from build123d import *

# Parameters (mm, degrees)
BOSS_EXTRUDE1_DEPTH = 13
SKETCH1_3_W         = 30
SKETCH1_3_H         = 13
BOSS_EXTRUDE2_DEPTH = 37
SKETCH2_R           = 8
CUT_EXTRUDE1_DEPTH  = 37


with BuildPart() as part:
    # Sketch1 → Boss-Extrude1 (new body)
    with BuildSketch(Plane(origin=(0, 0, 0), x_dir=(1, 0, 0), z_dir=(0, 1, 0))):
        with BuildLine():
            ThreePointArc((0, 30), (-15, 15), (0, 0))
            Line((0, 0), (0, 8.5))
            ThreePointArc((0, 8.5), (-6.5, 15), (0, 21.5))
            Line((0, 21.5), (0, 30))
        make_face()
        with BuildLine():
            Line((0, 8.5), (0, 0))
            ThreePointArc((0, 0), (10.606601718, 4.393398282), (15, 15))
            ThreePointArc((15, 15), (10.606601718, 25.606601718), (0, 30))
            Line((0, 30), (0, 21.5))
            ThreePointArc((0, 21.5), (4.596194078, 19.596194078), (6.5, 15))
            ThreePointArc((6.5, 15), (4.596194078, 10.403805922), (0, 8.5))
        make_face()
        with BuildLine():
            ThreePointArc((15, 15), (10.606601718, 4.393398282), (0, 0))
            Line((0, 0), (35, 0))
            Line((35, 0), (35, 30))
            Line((35, 30), (5, 30))
            Line((5, 30), (0, 30))
            ThreePointArc((0, 30), (10.606601718, 25.606601718), (15, 15))
        make_face()
    extrude(amount=BOSS_EXTRUDE1_DEPTH)

    # Sketch1_3 → Boss-Extrude2 (add)
    with BuildSketch(Plane(origin=(0, 0, 0), x_dir=(1, 0, 0), z_dir=(0, 1, 0))):
        with Locations((20, 36.5)):
            Rectangle(SKETCH1_3_W, SKETCH1_3_H)
    extrude(amount=BOSS_EXTRUDE2_DEPTH)

    # Sketch2 → Cut-Extrude1 (cut)
    with BuildSketch(Plane.XY.offset(-30)):
        with Locations((20, 25)):
            Circle(SKETCH2_R)
    extrude(amount=-CUT_EXTRUDE1_DEPTH, mode=Mode.SUBTRACT)


solid = part.part
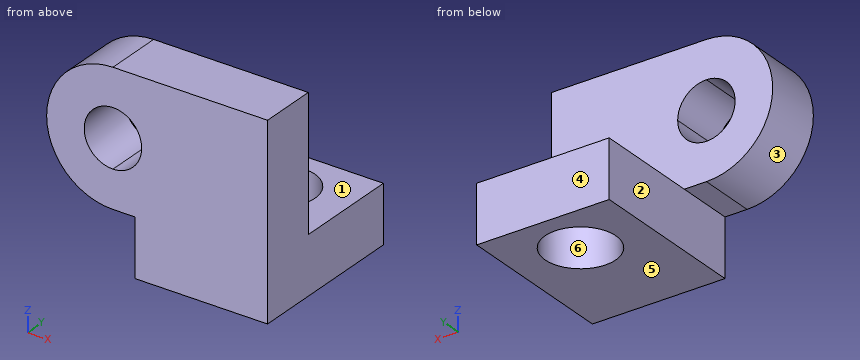
Part model, mm, in its own coordinate system. Face numbers are marked on the shaded views. A direction names the side the tool comes from. Coordinates: 2 decimals unless noted, no trailing zeros. Order: outer loops, then holes, each group sorted by start corner. A loop starts at its lowest first (then second) coordinate and runs counter-clockwise, first axis right, second up. Notation, with made-up numbers: M 63,23.5 L 112,23.5 A35 cw 112,60.5 Z; hole C 54,82.25 d5. An arc over 180 degrees is marked long. Use a Markdown table: item, result.
(1) Flat gauge pins, fed straight in: pin 1 (14.5 mm diameter, centred on x = 20, y = 25, fed in from +Z); pin 2 (10 mm diameter, centred on x = 2, y = 18.5, fed in from +Z); pin 3 (10 mm diameter, centred on x = 3, z = -19, fed in from +Y); pin 4 (6.5 mm diameter, centred on y = 16, z = -33.5, fed in from -X). Where does each tip first touch, or does it go through?
A:
| item | result |
|---|---|
| pin 1 | passes through |
| pin 2 | stops at z = -30 |
| pin 3 | stops at y = 13 |
| pin 4 | stops at x = 5 |
(2) Probe L1, parallel to Y at x = 20, z = -38; L2, parallel to Y at x = 4.5, z = -23; L3, parallel to Z at x = -2.5, y = 5. List the from-to ranges inside material, lowest first.
A:
| item | result |
|---|---|
| L1 | y = 0 to 17, 33 to 37 |
| L2 | y = 0 to 13 |
| L3 | z = -29.79 to -21, -9 to -0.21 |
(3) Cut at B-B on y = 7. Write the cut outline in (x, z), then the cut area to 3 significant figures.
A:
| item | result |
|---|---|
| outline | M 0,-30 L 5,-30 L 5,-43 L 35,-43 L 35,0 L 0,0 A15 ccw Z; hole C 0,-15 d13 |
| area | 1,660 mm^2 |
(4) Cut at A-A on x = 20. Write the cut outline in (y, z).
A:
| item | result |
|---|---|
| outline | M 0,-43 L 17,-43 L 17,-30 L 13,-30 L 13,0 L 0,0 Z; M 33,-43 L 37,-43 L 37,-30 L 33,-30 Z |
(5) Cut at D-D on x = 31.5. Write the cut outline in (y, z), then the cut area to 3 significant figures.
A:
| item | result |
|---|---|
| outline | M 0,-43 L 37,-43 L 37,-30 L 13,-30 L 13,0 L 0,0 Z |
| area | 871 mm^2 |
(6) Pull direction Y, two halves, no side cores. Call the marked faces 4, 5 and 6: released by +Y, released by -Y, zero draft, split by the parting line, or undercut.
A:
| item | result |
|---|---|
| face 4 | released by +Y |
| face 5 | zero draft |
| face 6 | undercut |
(7) Cut at C-C on z = -33. Write the cut outline in (x, y).
A:
| item | result |
|---|---|
| outline | M 5,0 L 35,0 L 35,37 L 5,37 Z; hole C 20,25 d16 |
(8) Tool access for the marked faces 1, 2 and 3: list every direction of +Z, -Z, +X, -X, +Y, -Y with a clear straight run to the whole face (end or side of a thin tool).
A:
| item | result |
|---|---|
| face 1 | +Z, +X, -X, +Y |
| face 2 | -Z, -X, +Y, -Y |
| face 3 | -X, +Y, -Y |
